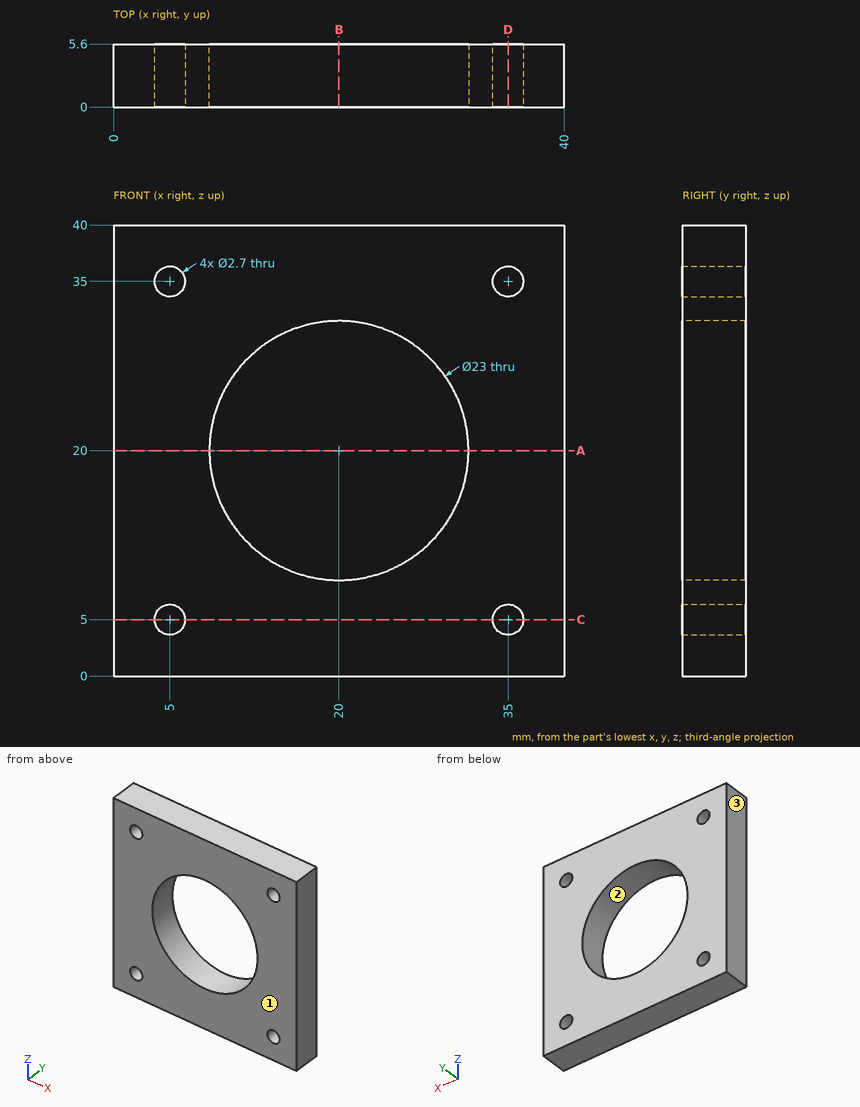
For this review, use the dimensioned drawing (mm, ordinates from the lowest corner) and the shaded views. Round coordinates to 2 decimals unless told otherwise and drop trailing zeros. Write each loop counter-clockwise with the first axis right and the second up, starting at its lowest first coordinate (ties: lowest second). Pieces come first, ordered by that corner, then holes. Notation, with made-up numbers: (63, 15.25) - (108, 15.25) arc R7 cw to (108, 24.25) - close; hole circle Ø4 at (82, 66). An arc over 180 degrees is marked (long way). One line per item, written item: value. Start each with the question number.
1. Consider section C-C on z = 5. Write out the cut boundary in (x, y).
2. Consider section A-A on z = 20. Write out the cut boundary in (x, y), and give its area (3 significant figures).
3. Consider section D-D on x = 35. Write out the cut boundary in (y, z).
4. Consider section B-B on x = 20. Write out the cut boundary in (y, z), and give its area (3 significant figures).
5. The part is to be moulded in two halves that separate along X. For the marked faces 1, 2 and 3, say which applies: released by +X, released by -X, zero draft, split by the parting line, or undercut.
6. To check wall thickness, follow L1, parallel to Z at x = 5, y = 1.7; L2, parallel to X at y = 1.9, z = 20. State the ranges of each line that lie inside material, in increasing order. Write a range as from..to.
7. Clearance check with a flat-ended pin moving along its axis: P1, Ø3, axis at x = 5, z = 5, coming from the -Y side. State where the tip first meets the part, or that it passes through.
Checks:
1. outline: (0, 0) - (3.65, 0) - (3.65, 5.6) - (0, 5.6) - close; (6.35, 0) - (33.65, 0) - (33.65, 5.6) - (6.35, 5.6) - close; (36.35, 0) - (40, 0) - (40, 5.6) - (36.35, 5.6) - close
2. outline: (0, 0) - (8.5, 0) - (8.5, 5.6) - (0, 5.6) - close; (31.5, 0) - (40, 0) - (40, 5.6) - (31.5, 5.6) - close
2. area: 95.2 mm^2
3. outline: (0, 0) - (5.6, 0) - (5.6, 3.65) - (0, 3.65) - close; (0, 6.35) - (5.6, 6.35) - (5.6, 33.65) - (0, 33.65) - close; (0, 36.35) - (5.6, 36.35) - (5.6, 40) - (0, 40) - close
4. outline: (0, 0) - (5.6, 0) - (5.6, 8.5) - (0, 8.5) - close; (0, 31.5) - (5.6, 31.5) - (5.6, 40) - (0, 40) - close
4. area: 95.2 mm^2
5. face 1: zero draft
5. face 2: undercut
5. face 3: released by -X
6. L1: z = 0..3.65, 6.35..33.65, 36.35..40
6. L2: x = 0..8.5, 31.5..40
7. P1: stops at y = 0
